Print and shaded views of the part. All mm, measured from the part's lowest x, y and z. Coordinates: 2 decimals unless noted, no trailing zeros. Order: outer loops, then holes, each group sorted by start corner. A loop starts at its lowest first (then second) coordinate and runs counter-clockwise, first axis right, second up. Notation, with made-up numbers: (21.5, 57) -> (26.5, 57) arc R11 cw to (26.5, 77) -> close; hole circle Ø4 at (-34.5, 24). An arc over 180 degrees is marked (long way). Return JSON: item names as keys, results as strings. Group by question number.
1) Cut at D-D (z = 34). Write the cut outline in (x, y), and give its area (3 significant figures).
2) Probe line 1 (X direction, y = 5.25, z = 133) (1 decimal); line 2 (X direction, y = 3.5, z = 131) (1 decimal); line 3 (Y direction, x = 15, z = 132.5). List the from-to ranges inside material, lowest first.
3) Flat gauge pin, fed straight in: pin 1 (7.5 mm diameter, centred on x = 133.35, z = 133.35, fed in from +Y). Where does the tip first touch, or does it go through?
4) Cut at A-A (y = 9.75). State how many separate pieces and enclosed holes the cut face has, and give its area (3 significant figures).
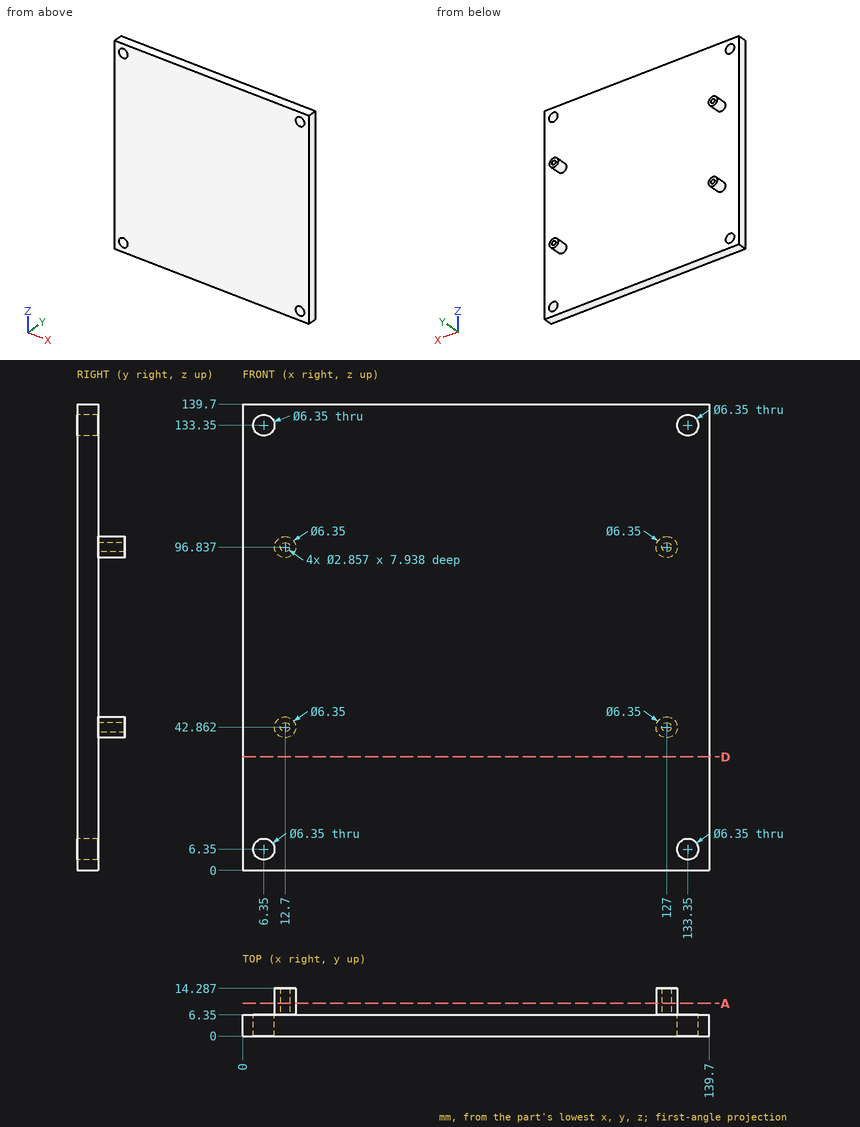
Answers below:
{
 "1": {"outline": "(0, 0) -> (139.7, 0) -> (139.7, 6.35) -> (0, 6.35) -> close", "area": "887 mm^2"},
 "2": {"line 1": "x = 0 to 3.2, 9.5 to 130.2, 136.5 to 139.7", "line 2": "x = 0 to 4.2, 8.5 to 131.2, 135.5 to 139.7", "line 3": "y = 0 to 6.35"},
 "3": {"pin 1": "stops at y = 6.35"},
 "4": {"separate pieces": "4", "enclosed holes": "4", "area": "101 mm^2"}
}
